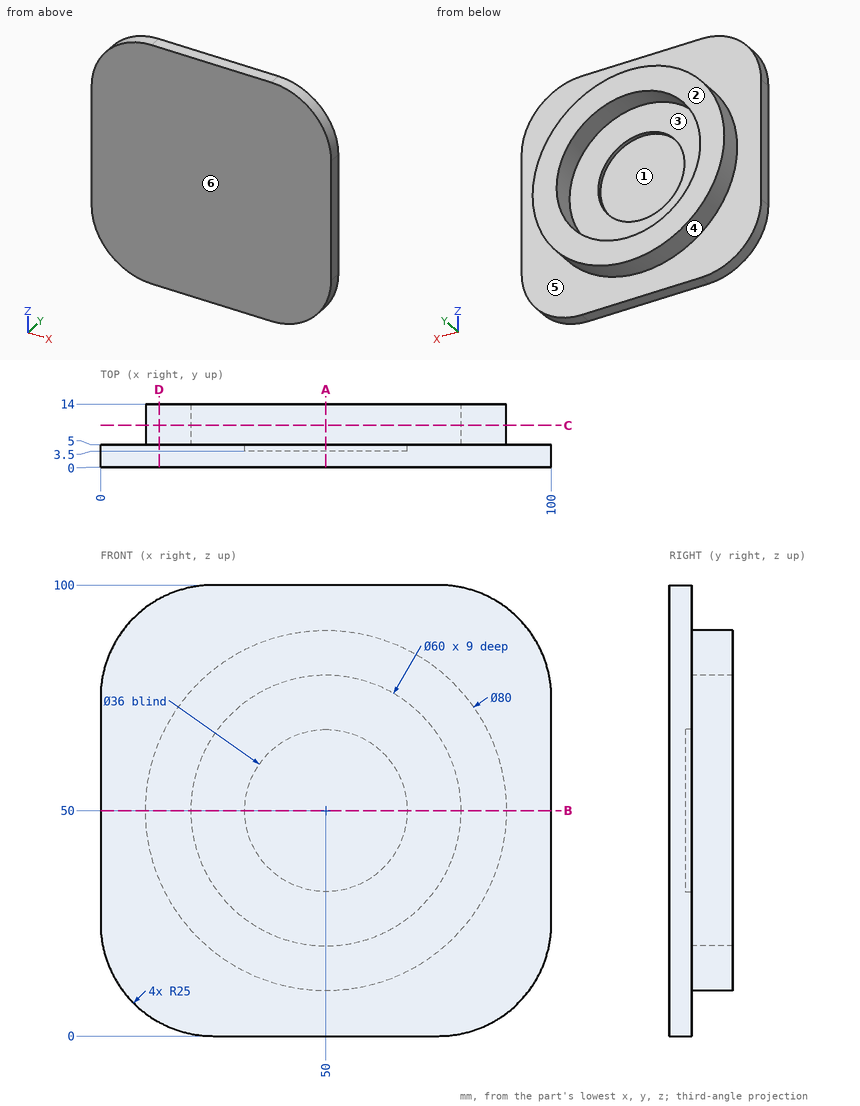
Study the drawing (mm; zero at the part's minimum x, y, z) and answer. A direction names the side the tool comes from. Coordinates: 2 decimals unless noted, no trailing zeros. Order: outer loops, then holes, each group sorted by start corner. A loop starts at its lowest first (then second) coordinate and runs counter-clockwise, first axis right, second up. Notation, with made-up numbers: M 20,54.5 L 41,54.5 A25 cw 41,75.5 Z; hole C 9,-29 d8. An arc over 180 degrees is marked long. Answer as a JSON object with one key per item and string values. Group by question number.
1. Section D-D on x = 13 is taken. Write down the section's boundary in (y, z).
2. Section B-B on z = 50 is taken. Write down the section's boundary in (x, y), then the cut area to 3 significant figures.
3. Determine the mould class of the marked faces 1, 2, 3 and 4 for opening direction Z: released by +Z, released by -Z, zero draft, split by the parting line, or undercut.
4. Straight lines are drawn through the part: line 1 (Z direction, x = 50, y = 7); line 2 (X direction, y = 4.4, z = 50). For each, find the intervals that lie inside material, in ascending order.
5. A tool of negligible diameter and unlimited length cuts with its end or side. For the marked faces 5 and 6, from which of +Z, -Z, +X, -X, +Y, -Y can it reach the whole face along a straight path? Write none if from no direction.
6. Flat-ended cylindrical pins translate along their axes: P1, Ø8, axis at x = 26.5, y = 11, coming from the +Z side; P2, Ø1.5, axis at x = 33.5, y = 8, coming from the -Z side; P3, Ø1.5, axis at x = 66.5, z = 74, coming from the +Y side. Find the tip coordinate at first contact, or state that the pin passes through.
7. Section A-A on x = 50 is taken. Write down the section's boundary in (y, z).
8. Section C-C on y = 9.25 is taken. Write down the section's boundary in (x, z), then the cut area to 3 significant figures.
Values follow:
{
 "1": {"outline": "M 0,3.07 L 5,3.07 L 5,34.8 L 14,34.8 L 14,65.2 L 5,65.2 L 5,96.93 L 0,96.93 Z"},
 "2": {"outline": "M 0,0 L 100,0 L 100,5 L 90,5 L 90,14 L 80,14 L 80,5 L 68,5 L 68,3.5 L 32,3.5 L 32,5 L 20,5 L 20,14 L 10,14 L 10,5 L 0,5 Z", "area": "626 mm2"},
 "3": {"face 1": "undercut", "face 2": "zero draft", "face 3": "undercut", "face 4": "split by the parting line"},
 "4": {"line 1": "10 to 20, 80 to 90", "line 2": "0 to 32, 68 to 100"},
 "5": {"face 5": "+Y", "face 6": "+Z, -Z, +X, -X, -Y"},
 "6": {"P1": "z = 84.92", "P2": "z = 13.23", "P3": "y = 5"},
 "7": {"outline": "M 0,0 L 5,0 L 5,10 L 14,10 L 14,20 L 5,20 L 5,32 L 3.5,32 L 3.5,68 L 5,68 L 5,80 L 14,80 L 14,90 L 5,90 L 5,100 L 0,100 Z"},
 "8": {"outline": "C 50,50 d80; hole C 50,50 d60", "area": "2,200 mm2"}
}
